Design review of the part built by this model. Coordinates are the model's own, in mm. Face numbers are marked on the shaded views. Give positions to 0.01 mm unless a question says otherwise; leave off trailing zeros. Loops run counter-clockwise (first coordinate to the right, second up) from the corner with the lowest first, then second, coordinate; pieces in that order, holes last. Notation, with made-up numbers: (-24.5, 5.25) -> (-1.5, 5.25) arc R28 ccw to (-1.5, 28.25) -> close; hole circle Ø7 at (-30.75, -2.5). An arc over 180 degrees is marked (long way). Answer in a Markdown table with one row per item. Add a question column.
(1) For line 1 (X direction, y = 1.05, z = 0); line 2 (Z direction, x = -32, y = 5.75); line 3 (Y direction, x = -30.5, z = -26), list the stretches that pass through material, from the lowest coordinate up.
(2) Draft analysis for pull direction X (two halves, no side actions). For the marked faces 1 and 2, state which applies: +X half, -X half, draft (parallel to the pull), parting line (faces both ways), or undercut.
(3) For pin 1 (7 mm diameter, centred on x = -22, z = 0, fed in from +Y); pin 2 (4 mm diameter, centred on y = 5.5, z = -7.5, fed in from +X); pin 3 (1.5 mm diameter, centred on x = 25, y = 5.5, fed in from -Z), all flat-tipped, find the tip position at first contact; note any pin that passes through.
(4) Consider section B-B on x = 0. Write out the cut boundary in (y, z), then the cut area to 3 significant figures.
(5) Consider section A-A on z = 0. Count the separate pieces of the cut face and the enclosed holes in it, then the cut area to 3 significant figures.
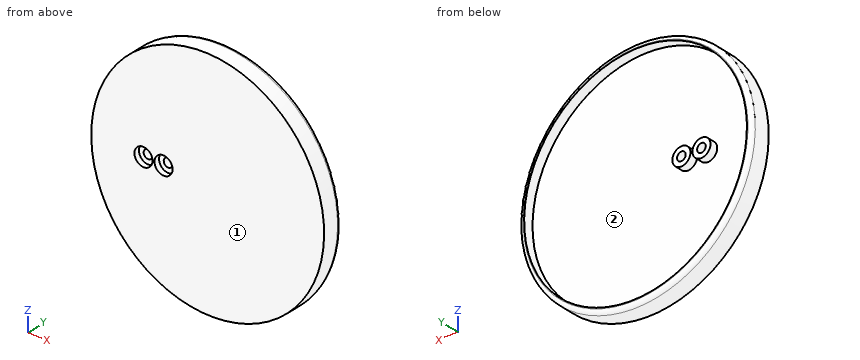
from build123d import *

# Parameters (mm, degrees)
SKETCH_1_R                            = 4.5
MOVING_POST_A_DEPTH                   = 9
SKETCH_2_R                            = 58
CUP_PLATE_D116_T5_DEPTH               = 5
SKETCH_3_R                            = 4.5
MOVING_POST_B_DEPTH                   = 9
SKETCH_4_R                            = 58
SKETCH_4_R_2                          = 55.5
DRIP_SKIRT_OD116_ID111_H10_DEPTH      = 10
SKETCH_5_R                            = 2.15
M4_MOVING_MOUNT_CLEARANCE_DEPTH       = 9
SKETCH_6_R                            = 4.5
M4_MOVING_HEAD_RECESS_D8P2_T2P7_DEPTH = 2.7
CUP_TOP_OUTER_ROUND_R2_R              = 2


with BuildPart() as part:
    # 草图1 → Moving_post_A (new body)
    with BuildSketch(Plane(origin=(0, 0, 0), x_dir=(1, 0, 0), z_dir=(0, 1, 0))):
        with Locations(Location((-22, 0, 0), (0, 0, 270))):
            Circle(SKETCH_1_R)
    extrude(amount=MOVING_POST_A_DEPTH)

    # 草图2 → Cup_plate_D116_T5 (add)
    with BuildSketch(Plane(origin=(0, 0, 0), x_dir=(1, 0, 0), z_dir=(0, 1, 0))):
        with Locations(Location((0, 0, 0), (0, 0, 270))):
            Circle(SKETCH_2_R)
    extrude(amount=CUP_PLATE_D116_T5_DEPTH)

    # 草图3 → Moving_post_B (add)
    with BuildSketch(Plane(origin=(0, 0, 0), x_dir=(1, 0, 0), z_dir=(0, 1, 0))):
        with Locations(Location((-32, 0, 0), (0, 0, 270))):
            Circle(SKETCH_3_R)
    extrude(amount=MOVING_POST_B_DEPTH)

    # 草图4 → Drip_skirt_OD116_ID111_H10 (add)
    with BuildSketch(Plane(origin=(0, 0, 0), x_dir=(1, 0, 0), z_dir=(0, 1, 0))):
        with Locations(Location((0, 0, 0), (0, 0, 270))):
            Circle(SKETCH_4_R)
        with Locations(Location((0, 0, 0), (0, 0, 270))):
            Circle(SKETCH_4_R_2, mode=Mode.SUBTRACT)
    extrude(amount=DRIP_SKIRT_OD116_ID111_H10_DEPTH)

    # 草图5 → M4_moving_mount_clearance (cut)
    with BuildSketch(Plane(origin=(0, 0, 0), x_dir=(1, 0, 0), z_dir=(0, 1, 0))):
        with Locations(Location((-22, 0, 0), (0, 0, 270))):
            Circle(SKETCH_5_R)
        with Locations(Location((-32, 0, 0), (0, 0, 270))):
            Circle(SKETCH_5_R)
    extrude(amount=M4_MOVING_MOUNT_CLEARANCE_DEPTH, mode=Mode.SUBTRACT)

    # 草图6 → M4_moving_head_recess_D8p2_T2p7 (cut)
    with BuildSketch(Plane(origin=(0, 0, 0), x_dir=(1, 0, 0), z_dir=(0, 1, 0))):
        with Locations(Location((-22, 0, 0), (0, 0, 270))):
            Circle(SKETCH_6_R)
        with Locations(Location((-32, 0, 0), (0, 0, 270))):
            Circle(SKETCH_6_R)
    extrude(amount=M4_MOVING_HEAD_RECESS_D8P2_T2P7_DEPTH, mode=Mode.SUBTRACT)

    # Cup_top_outer_round_R2
    cup_top_outer_round_r2_edges = [part.edges().sort_by_distance(p)[0] for p in [
        (0, 10, -58),
    ]]
    fillet(cup_top_outer_round_r2_edges, radius=CUP_TOP_OUTER_ROUND_R2_R)


solid = part.part
Values follow:
| question | item | result |
|---|---|---|
| 1 | line 1 | -58 to -36.5, -27.5 to -26.5, -17.5 to 58 |
| 1 | line 2 | -48.37 to -45.35, -4.5 to -2.15, 2.15 to 4.5, 45.35 to 48.37 |
| 1 | line 3 | 0 to 5 |
| 2 | face 1 | draft |
| 2 | face 2 | undercut |
| 3 | pin 1 | y = 9 |
| 3 | pin 2 | x = 57.74 |
| 3 | pin 3 | z = -52.69 |
| 4 | outline | (0, -58) -> (8, -58) arc R2 ccw to (10, -56) -> (10, -55.5) -> (5, -55.5) -> (5, 55.5) -> (10, 55.5) -> (10, 56) arc R2 ccw to (8, 58) -> (0, 58) -> close |
| 4 | area | 603 mm2 |
| 5 | separate pieces | 3 |
| 5 | enclosed holes | 0 |
| 5 | area | 573 mm2 |
